Job drawing, mm, ordinate dimensions from the low corner. One solid piece. Round coordinates to 2 decimals unless told otherwise and drop trailing zeros. Write each loop counter-clockwise with the first axis right and the second up, starting at its lowest first coordinate (ties: lowest second). Pieces come first, ordered by that corner, then holes.
1) Flat gauge pins, fed straight in: pin 1 (15 mm diameter, centred on x = 273, y = 6.5, fed in from -Z); pin 2 (5.5 mm diameter, centred on x = 176, y = 17.5, fed in from +Z) (3 decimals). Where does each tip first touch, or does it go through?
2) Saw through at B-B (x = 145.5). Write the cut outline in (y, z) (3 decimals).
3) Saw through at A-A (z = 13.5). Write the cut outline in (x, y).
4) Pull direction X, two halves, no side cores. Call the marked faces 1, 2, 3 and 4: +X half, -X half, draft (parallel to the pull), parting line (faces both ways), or undercut.
5) Wall check: probe 1 along X at (y, z) = (9.5, 59.5); probe 2 along Z at (x, y) = (102, 21) (3 decimals); probe 3 along Y at (x, z) = (259, 74). Give the ranges that are in metal, low to high.
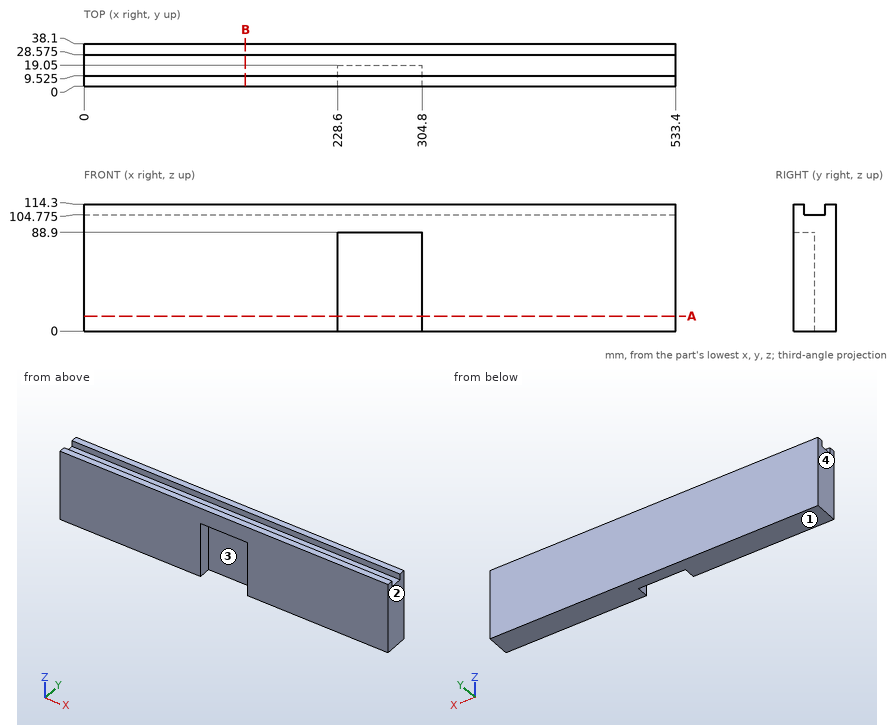
Evaluation:
1. pin 1: stops at z = 88.9
1. pin 2: stops at z = 104.775
2. outline: (0, 0) - (38.1, 0) - (38.1, 114.3) - (28.575, 114.3) - (28.575, 104.775) - (9.525, 104.775) - (9.525, 114.3) - (0, 114.3) - close
3. outline: (0, 0) - (228.6, 0) - (228.6, 19.05) - (304.8, 19.05) - (304.8, 0) - (533.4, 0) - (533.4, 38.1) - (0, 38.1) - close
4. face 1: draft
4. face 2: +X half
4. face 3: undercut
4. face 4: -X half
5. probe 1: x = 0 to 228.6, 304.8 to 533.4
5. probe 2: z = 0 to 104.775
5. probe 3: y = 19.05 to 38.1
